Geometry check sheet. Reference: the model listing, model coordinates, mm. A direction names the side the tool comes from. Give positions to 0.01 mm unless a question says otherwise; leave off trailing zeros. Order: outer loops, then holes, each group sorted by start corner. A loop starts at its lowest first (then second) coordinate and runs counter-clockwise, first axis right, second up. Notation, with made-up numbers: M 89,9 L 144,9 A24 ccw 144,37 Z; hole C 64,-37 d1. An arc over 180 degrees is marked long. Answer as CSV lines item,"result". Start each with the question number.
Q1. Mould release check, pull along X, two halves, no side actions. Record for faces 1 (the cylindrical face through (0.303, -46.954, -4.637)), 2 (the flat face through (-19.05, -35, 0)), 3 (the cylindrical face through (1.07, -15.12, -11.59)): +X half, -X half, draft (parallel to the pull), parting line (faces both ways), or undercut.
Q2. Section check B-B, the plane y = 0. Record the boundary of the cut face in (x, z) (3 decimals), then the cut area to 3 significant figures.
Q3. Go/stop test with flat-tipped pins: pin 1 (15 mm diameter, centred on x = 3.5, y = -33, fed in from +Z); pin 2 (4 mm diameter, centred on x = -33.5, z = -9, fed in from -Y); pin 3 (1.5 mm diameter, centred on x = 27, z = -33, fed in from +Y); pin 4 (12 mm diameter, centred on y = -8.5, z = -38, fed in from -X). Record where each tip stops, or that it passes through.
Q4. Thickness scan on line 1 (Z direction, x = -27.5, y = 0) (3 decimals); line 2 (Z direction, x = 6.35, y = -47.6) (3 decimals); line 3 (Y direction, x = 20, z = -42.5). Record the ranges inside material, lowest first.
Q5. Set-up check for faces 4 (the flat face through (0, -35, 12.7)), 5 (the flat face through (50.8, -24, -1)), 6 (the flat face through (-1, -19.05, 43)), 7 (the flat face through (-50.8, -24, -1)): record each of +Z, -Z, +X, -X, +Y, -Y from which the full face is reachable in a straight line by a thin tool's end or side.
Q6. Section check C-C, the plane x = 3. Record the boundary of the cut face in (y, z) (3 decimals), then the cut area to 3 significant figures.
Q7. Section check A-A, the plane z = 0. Record the boundary of the cut face in (x, y) (3 decimals).
Q8. Section check D-D, the plane x = -22.5. Record the boundary of the cut face in (y, z) (3 decimals).
```python
from build123d import *

# Parameters (mm, degrees)
F0_R          = 22.225
F1_DEPTH      = 76.2
F1_DEPTH_BACK = 76.2
F3_START      = 19.05
F2_W          = 101.6
F2_H          = 101.6
F3_DEPTH      = 6.35
F4_R          = 12.7
F5_W          = 38.1
F5_H          = 25.4
F6_DEPTH      = 19.05
F7_R          = 9.525
F7_R_2        = 7.62
F8_DEPTH      = 5.08
F9_R          = 19.05
F10_DEPTH     = 152.4


with BuildPart() as f1:
    # F0 (on Right) → F1 (new body, two sides)
    with BuildSketch(Plane.YZ) as f1_sk:
        Circle(F0_R)
    extrude(amount=F1_DEPTH)
    extrude(f1_sk.sketch, amount=-F1_DEPTH_BACK)

    # F2 (on Front) → F3 (join)
    with BuildSketch(Plane.XZ.offset(F3_START)):
        Rectangle(F2_W, F2_H)
    extrude(amount=F3_DEPTH)

    # F4
    f4_edges = [f1.edges().sort_by_distance(p)[0] for p in [
        (0, -19.05, 11.447625),
        (0, -19.05, -11.447625),
    ]]
    fillet(f4_edges, radius=F4_R)

    # F5 (on face) → F6 (join)
    with BuildSketch(Plane.XZ.offset(25.4)):
        Rectangle(F5_W, F5_H)
    extrude(amount=F6_DEPTH)

    # F7 (on face) → F8 (join)
    with BuildSketch(Plane.XZ.offset(44.45)):
        with Locations((6.35, 0)):
            Circle(F7_R)
        with Locations((6.35, 0)):
            Circle(F7_R_2, mode=Mode.SUBTRACT)
    extrude(amount=F8_DEPTH)

    # F9 (on face) → F10 (cut)
    with BuildSketch(Plane.YZ.offset(76.2)):
        Circle(F9_R)
    extrude(amount=-F10_DEPTH, mode=Mode.SUBTRACT)


solid = f1.part
```
Answer block:
1,face 1,"undercut"
1,face 2,"-X half"
1,face 3,"draft"
2,outline,"M -76.2,-22.225 L 76.2,-22.225 L 76.2,-19.05 L -76.2,-19.05 Z; M -76.2,19.05 L 76.2,19.05 L 76.2,22.225 L -76.2,22.225 Z"
2,area,"968 mm2"
3,pin 1,"stops at z = 12.7"
3,pin 2,"stops at y = -25.4"
3,pin 3,"stops at y = -18.88"
3,pin 4,"passes through"
4,line 1,"z = -22.225 to -19.05, 19.05 to 22.225"
4,line 2,"z = -9.525 to -7.62, 7.62 to 9.525"
4,line 3,"y = -25.4 to -19.05"
5,face 4,"+Z, +X, -X, -Y"
5,face 5,"+X, -Y"
5,face 6,"+Z, +X, -X, +Y"
5,face 7,"-X, -Y"
6,outline,"M -49.53,-8.916 L -44.45,-8.916 L -44.45,-12.7 L -25.4,-12.7 L -25.4,-50.8 L -19.05,-50.8 L -19.05,-34.343 A12.7 cw -4.041,-21.855 A22.225 ccw long -4.041,21.855 A12.7 cw -19.05,34.343 L -19.05,50.8 L -25.4,50.8 L -25.4,12.7 L -44.45,12.7 L -44.45,8.916 L -49.53,8.916 L -49.53,6.844 L -44.45,6.844 L -44.45,-6.844 L -49.53,-6.844 Z; hole C 0,0 d38.1"
6,area,"1,680 mm2"
7,outline,"M -76.2,-22.225 L -50.8,-22.225 L -50.8,-25.4 L -19.05,-25.4 L -19.05,-44.45 L -3.175,-44.45 L -3.175,-49.53 L -1.27,-49.53 L -1.27,-44.45 L 13.97,-44.45 L 13.97,-49.53 L 15.875,-49.53 L 15.875,-44.45 L 19.05,-44.45 L 19.05,-25.4 L 50.8,-25.4 L 50.8,-22.225 L 76.2,-22.225 L 76.2,-19.05 L -76.2,-19.05 Z; M -76.2,19.05 L 76.2,19.05 L 76.2,22.225 L -76.2,22.225 Z"
8,outline,"M -25.4,-50.8 L -19.05,-50.8 L -19.05,-34.343 A12.7 cw -4.041,-21.855 A22.225 ccw long -4.041,21.855 A12.7 cw -19.05,34.343 L -19.05,50.8 L -25.4,50.8 Z; hole C 0,0 d38.1"
